from build123d import *


with BuildPart() as part:
    # Sketch1 → Revolve1 (revolve)
    with BuildSketch(Plane(origin=(0, 0, 0), x_dir=(-1, 0, 0), z_dir=(0, 1, 0))):
        with BuildLine():
            Line((-1, 10), (-3.5, 10))
            Line((-3.5, 10), (-4.5, 9))
            Line((-4.5, 9), (-4.5, 0))
            Line((-4.5, 0), (23.5, 0))
            Line((23.5, 0), (23.5, 5))
            Line((23.5, 5), (22.5, 6))
            Line((22.5, 6), (21.6, 6))
            ThreePointArc((21.6, 6), (21.387867966, 5.912132034), (21.3, 5.7))
            Line((21.3, 5.7), (21.3, 5.5))
            ThreePointArc((21.3, 5.5), (21.212132034, 5.287867966), (21, 5.2))
            Line((21, 5.2), (20.3, 5.2))
            ThreePointArc((20.3, 5.2), (20.087867966, 5.287867966), (20, 5.5))
            Line((20, 5.5), (20, 5.7))
            ThreePointArc((20, 5.7), (19.912132034, 5.912132034), (19.7, 6))
            Line((19.7, 6), (2, 6))
            ThreePointArc((2, 6), (0.585786438, 6.585786438), (0, 8))
            Line((0, 8), (0, 9))
            Line((0, 9), (-1, 10))
        make_face()
    revolve(axis=Axis((-23.5, 0, 0), (1, 0, 0)))


solid = part.part
Read the model definition and answer for the solid it produces. Units are mm, in the model's axes. A direction names the side the tool comes from. Give positions to 0.01 mm unless a question says otherwise; leave off trailing zeros. Return JSON: item names as keys, results as strings.
Q1. Given P1, Ø3, axis at x = -11, y = 5.5, coming from the +Z side; P2, Ø8, axis at x = -3.5, y = 6, coming from the -Z side; P3, Ø6, axis at y = -7, z = -8, coming from the -X side, each flat-ended and moving along its own axis, determine where each tip first touches the part or whether it passes through.
Reply:
{"P1": "z = 4.47", "P2": "z = -8.04", "P3": "x = -0.03"}
Q2. For a pull along X with two mould halves and no side action, classify faces 3 (the face through (-23.5, 0, 0)), 4 (the face through (4.5, 0, 0)), 5 (the face through (-20.645, -5.156, -0.677)) as released by +X, released by -X, zero draft, split by the parting line, or undercut.
Reply:
{"face 3": "released by -X", "face 4": "released by +X", "face 5": "undercut"}
Q3. Consider line 1 along Y through (x, z) = (-15.5, 0); line 2 along X through (y, z) = (6, -5.25); line 3 along X through (y, z) = (-5.25, -0.75). Determine where each line is inside the solid, lowest interval first. Write a range as [from, to].
Reply:
{"line 1": "[-6, 6]", "line 2": "[0, 4.5]", "line 3": "[-23.2, -21.23], [-20.07, 4.5]"}
Q4. For faces 1 (the face through (-11, 0, -6)), 2 (the face through (2.27, 9.76, -2.17)), determine the directions among +Z, -Z, +X, -X, +Y, -Y from which every point of the face is accessible in a straight line to the end or side of a thin tool.
Reply:
{"face 1": "-X", "face 2": "+X, -X"}
